from build123d import *

# Parameters (mm, degrees)
SKETCH1_W                                     = 340
SKETCH1_H                                     = 150
VERTICAL_PORTION_DEPTH                        = 10
SHAFT_ADAPTER_RIGHT_DEPTH                     = 25
SHAFT_ADAPTER_FILLETS_R                       = 5
SKETCH5_W                                     = 100
SKETCH5_H                                     = 5
LIMIT_TAB_PREVENTS_GATE_FROM_GETTING_PU_DEPTH = 10
LIMIT_TAB_FILLETS_R                           = 5


with BuildPart() as part:
    # Sketch1 → Vertical portion (new body)
    with BuildSketch(Plane.XY):
        Rectangle(SKETCH1_W, SKETCH1_H)
    extrude(amount=VERTICAL_PORTION_DEPTH)

    # Sketch4 → Shaft adapter right (add)
    with BuildSketch(Plane(origin=(155, 0, 0), x_dir=(0, 0, -1), z_dir=(1, 0, 0))):
        with BuildLine():
            Line((-10, 45), (-30, 52.5))
            Line((-30, 52.5), (-30, 60))
            Line((-30, 60), (-25, 60))
            ThreePointArc((-25, 60), (-20, 55), (-15, 60))
            Line((-15, 60), (-10, 60))
            Line((-10, 60), (-10, 55))
            Line((-10, 55), (-10, 45))
        make_face()
    shaft_adapter_right = extrude(amount=-SHAFT_ADAPTER_RIGHT_DEPTH)

    # Shaft adapter left: Shaft adapter right across plane
    add(shaft_adapter_right.mirror(Plane(origin=(0, 0, 0), x_dir=(0, 0, 1), z_dir=(1, 0, 0))))

    # Shaft adapter fillets
    shaft_adapter_fillets_edges = [part.edges().sort_by_distance(p)[0] for p in [
        (-142.5, 52.5, 30),
        (142.5, 52.5, 30),
        (130, 52.5, 10),
        (-130, 52.5, 10),
        (-142.5, 45, 10),
        (142.5, 45, 10),
        (142.5, 60, 10),
        (-142.5, 60, 10),
    ]]
    fillet(shaft_adapter_fillets_edges, radius=SHAFT_ADAPTER_FILLETS_R - 0.0001)  # a hair under: the kernel refuses the full size

    # Sketch5 → Limit tab (prevents gate from getting pushed out of slot) (add)
    with BuildSketch(Plane(origin=(0, 0, 0), x_dir=(-1, 0, 0), z_dir=(0, 0, -1))):
        with Locations((-100, -72.5)):
            Rectangle(SKETCH5_W, SKETCH5_H)
        with Locations((100, -72.5)):
            Rectangle(SKETCH5_W, SKETCH5_H)
    extrude(amount=LIMIT_TAB_PREVENTS_GATE_FROM_GETTING_PU_DEPTH)

    # Limit tab fillets
    limit_tab_fillets_edges = [part.edges().sort_by_distance(p)[0] for p in [
        (150, -72.5, 0),
        (50, -72.5, 0),
        (100, -70, 0),
        (-150, -72.5, 0),
        (-100, -70, 0),
        (-50, -72.5, 0),
    ]]
    fillet(limit_tab_fillets_edges, radius=LIMIT_TAB_FILLETS_R)


solid = part.part
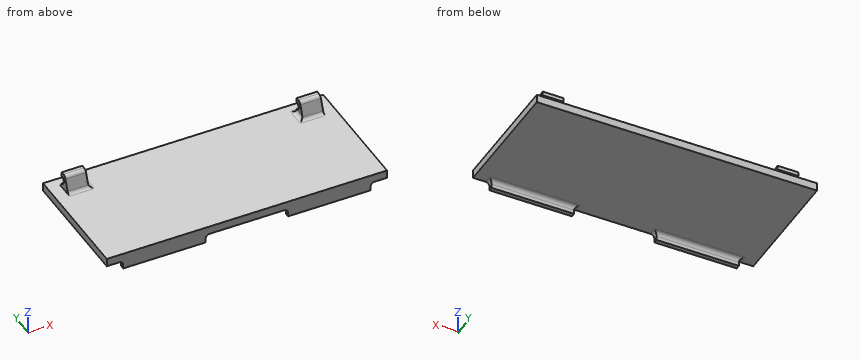
The listing builds one solid part. Answer for the finished solid, in the listing's coordinates (mm). Give positions to 0.01 mm unless a question says otherwise; leave off trailing zeros. Loops run counter-clockwise (first coordinate to the right, second up) from the corner with the lowest first, then second, coordinate; pieces in that order, holes last. Notation, with made-up numbers: (-36, -20) - (-10, -20) arc R27 cw to (-10, 3) - close; hole circle Ø11 at (1, 61.25). An arc over 180 degrees is marked (long way). Write each question's results on one line, items separated by ' | '.
1. Find section A-A, the plane z = 20. Write down the section's boundary in (x, y), then the cut area to 4 significant figures.
Resolved:
outline: (-155, 48.75) - (-130, 48.75) - (-130, 55) - (-155, 55) - close; (130, 48.75) - (155, 48.75) - (155, 55) - (130, 55) - close | area: 312.5 mm^2
2. Find section C-C, the plane x = -40.5. Write down the section's boundary in (y, z).
Resolved:
outline: (-75, 0) - (75, 0) - (75, 10) - (-75, 10) - close
3. Flat-ended cylindrical pins translate along their axes: P1, Ø6.5, axis at y = 50.5, z = 23.5, coming from the -X side; P2, Ø3, axis at x = -16.5, y = -45.5, coming from the +Z side; P3, Ø2.5, axis at x = -141, z = 28.5, coming from the +Y side. Find the tip coordinate at first contact, or state that the pin passes through.
Resolved:
P1: stops at x = -155 | P2: stops at z = 10 | P3: stops at y = 60
4. Consider probe 1 along Z at (x, y) = (0, 43); probe 2 along X at (y, z) = (48, 13.5); probe 3 along Y at (x, z) = (-147, 11). Determine where each line is inside the solid, lowest interval first. Write a range as from..to.
Resolved:
probe 1: z = 0..10 | probe 2: x = -155..-129.77, 129.77..155 | probe 3: y = 44.54..62
5. Find section B-B, the plane y = -30.5. Write down the section's boundary in (x, z), then the cut area to 3 significant figures.
Resolved:
outline: (-170, 0) - (170, 0) - (170, 10) - (-170, 10) - close | area: 3,400 mm^2
